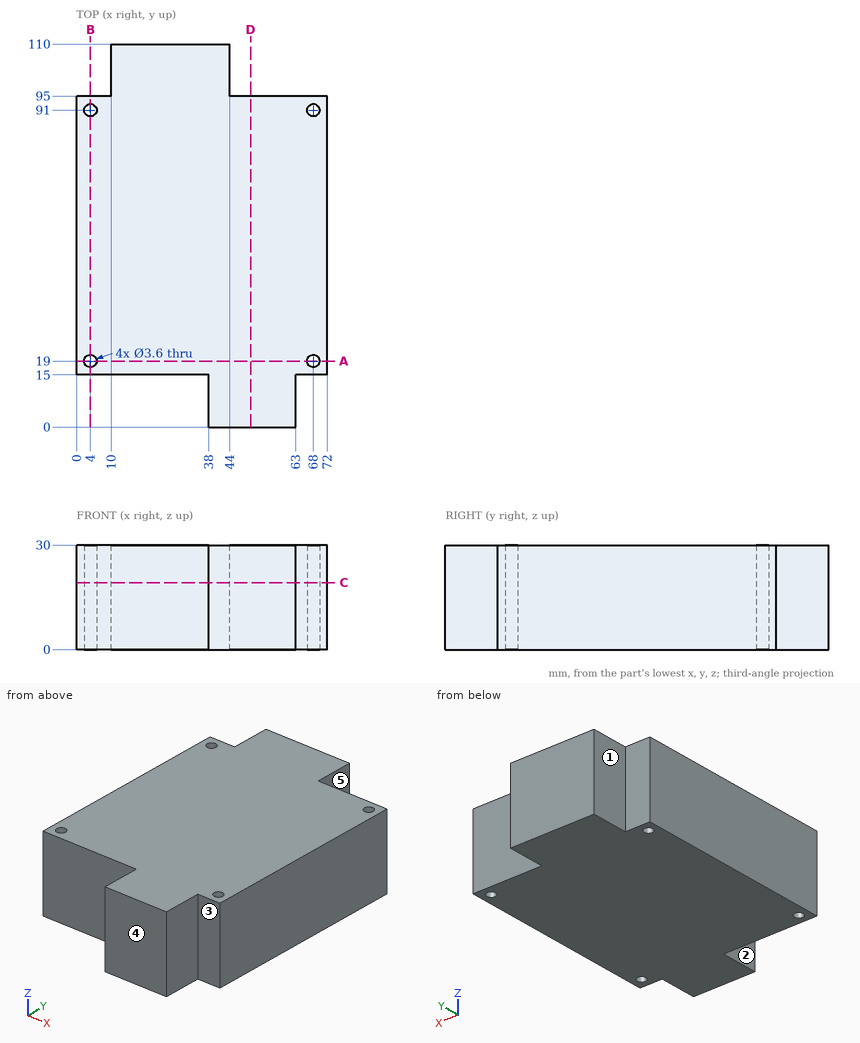
Could you check a few things on this drawing? It's one solid part, dimensions in mm from its lowest x, y, z. A direction names the side the tool comes from. Coordinates: 2 decimals unless noted, no trailing zeros. Loops run counter-clockwise (first coordinate to the right, second up) from the corner with the lowest first, then second, coordinate; pieces in that order, holes last.
1. For P1, Ø4.5, axis at x = 68.5, z = 21, coming from the -Y side; P2, Ø8, axis at x = 3.5, z = 18.5, coming from the +Y side; P3, Ø7.5, axis at y = 6, z = 15.5, coming from the -X side, each with a flat end and sliding along its axis, tell me the tip position at first contact or that it passes through.
2. Imagine slicing it at A-A (y = 19). Please give me the cut outline in (x, z).
3. Imagine slicing it at B-B (x = 4). Please give me the cut outline in (y, z).
4. Imagine slicing it at D-D (x = 50). Please give me the cut outline in (y, z).
5. I need wall thicknesses on L1, parallel to X at y = 91, z = 13.5; L2, parallel to Y at x = 4, z = 23; L3, parallel to Y at x = 36, z = 9. Which ranges of each line are inside material? Lowest first, please.
6. Imagine slicing it at C-C (z = 19.25). Please give me the cut outline in (x, y).
7. For the marked faces 1, 2, 3, 4 and 5, which set-ups out of +Z, -Z, +X, -X, +Y, -Y let a thin tool reach every point of the face, with its end or its side?
Computed values:
1. P1: stops at y = 15
1. P2: stops at y = 95
1. P3: stops at x = 38
2. outline: (0, 0) - (2.2, 0) - (2.2, 30) - (0, 30) - close; (5.8, 0) - (66.2, 0) - (66.2, 30) - (5.8, 30) - close; (69.8, 0) - (72, 0) - (72, 30) - (69.8, 30) - close
3. outline: (15, 0) - (17.2, 0) - (17.2, 30) - (15, 30) - close; (20.8, 0) - (89.2, 0) - (89.2, 30) - (20.8, 30) - close; (92.8, 0) - (95, 0) - (95, 30) - (92.8, 30) - close
4. outline: (0, 0) - (95, 0) - (95, 30) - (0, 30) - close
5. L1: x = 0 to 2.2, 5.8 to 66.2, 69.8 to 72
5. L2: y = 15 to 17.2, 20.8 to 89.2, 92.8 to 95
5. L3: y = 15 to 110
6. outline: (0, 15) - (38, 15) - (38, 0) - (63, 0) - (63, 15) - (72, 15) - (72, 95) - (44, 95) - (44, 110) - (10, 110) - (10, 95) - (0, 95) - close; hole circle Ø3.6 at (4, 19); hole circle Ø3.6 at (4, 91); hole circle Ø3.6 at (68, 19); hole circle Ø3.6 at (68, 91)
7. face 1: +Z, -Z, -X, +Y
7. face 2: +Z, -Z, -X, -Y
7. face 3: +Z, -Z, +X, -Y
7. face 4: +Z, -Z, +X, -X, -Y
7. face 5: +Z, -Z, +X, +Y
